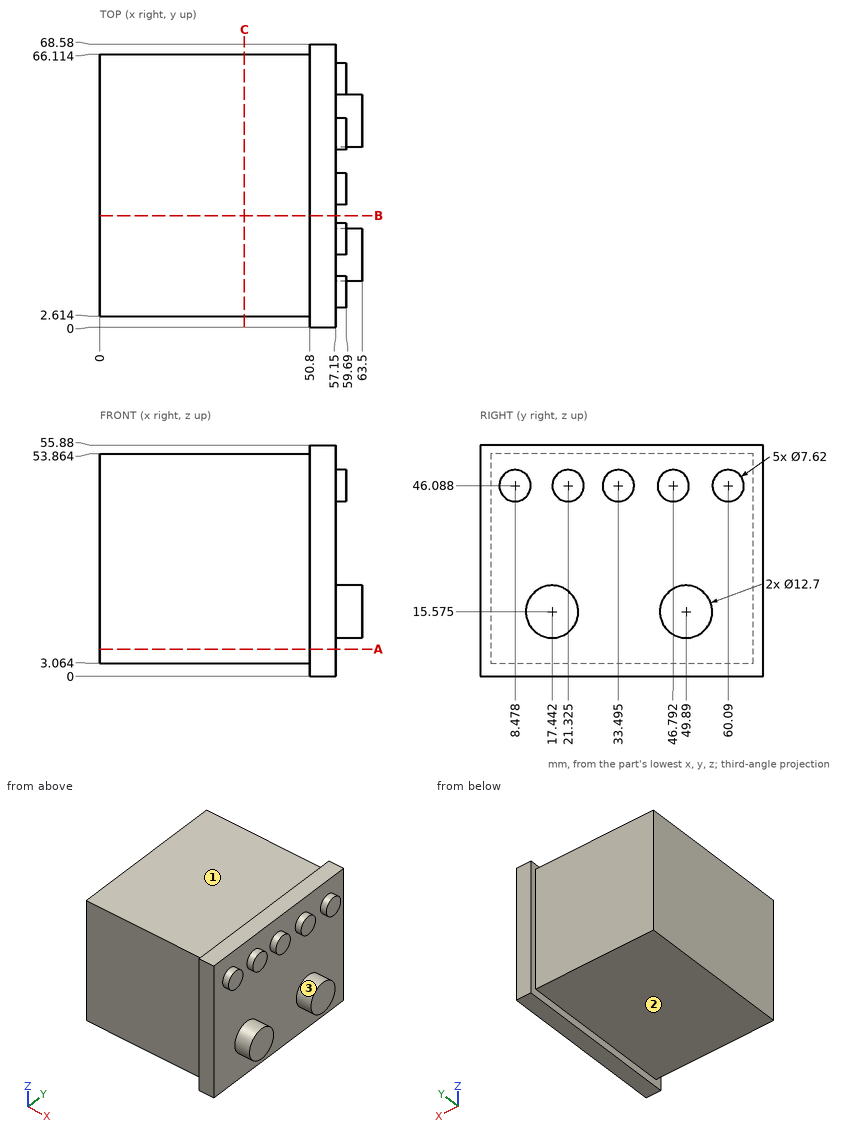
Input: dimensioned drawing with shaded views. Units: mm. Origin: part minimum x, y, z. A direction names the side the tool comes from. Give positions to 0.01 mm unless a question says otherwise; leave off trailing zeros. Write each loop counter-clockwise with the first axis right and the second up, starting at its lowest first coordinate (ties: lowest second). Pieces come first, ordered by that corner, then holes.
Q1. Section B-B, the plane y = 27. Output: boundary loops of the cut face in (x, z), plus the area to 3 significant figures.
Q2. First-contact query: P1, Ø1.5, axis at y = 28.5, z = 21.5, coming from the +X side; P2, Ø3, axis at x = 19.5, y = 38, coming from the +Z side; P3, Ø8.5, axis at y = 46, z = 47.5, coming from the +X side. Flat tips, straight axial feed; report the tip coordinate or a pass-through.
Q3. Material intervals for probe 1 along Z at (x, y) = (34.5, 64); probe 2 along Y at (x, z) = (18, 32.5); probe 3 along X at (y, z) = (33.5, 51), sorted ascending.
Q4. Section A-A, the plane z = 6.5. Output: boundary loops of the cut face in (x, y).
Q5. Section C-C, the plane x = 35. Output: boundary loops of the cut face in (y, z), plus the area to 3 significant figures.
Q6. Set-up query: the marked faces 1, 2 and 3. Return all of +Z, -Z, +X, -X, +Y, -Y with unobstructed straight access to the full face (end or side cutting, diameter ignored); none if empty.
Filled in:
1. outline: (0, 3.06) - (50.8, 3.06) - (50.8, 0) - (57.15, 0) - (57.15, 55.88) - (50.8, 55.88) - (50.8, 53.86) - (0, 53.86) - close
1. area: 2,940 mm2
2. P1: stops at x = 57.15
2. P2: stops at z = 53.86
2. P3: stops at x = 59.69
3. probe 1: z = 3.06 to 53.86
3. probe 2: y = 2.61 to 66.11
3. probe 3: x = 0 to 57.15
4. outline: (0, 2.61) - (50.8, 2.61) - (50.8, 0) - (57.15, 0) - (57.15, 68.58) - (50.8, 68.58) - (50.8, 66.11) - (0, 66.11) - close
5. outline: (2.61, 3.06) - (66.11, 3.06) - (66.11, 53.86) - (2.61, 53.86) - close
5. area: 3,230 mm2
6. face 1: +Z, -X, +Y, -Y
6. face 2: -Z, -X, +Y, -Y
6. face 3: +X
